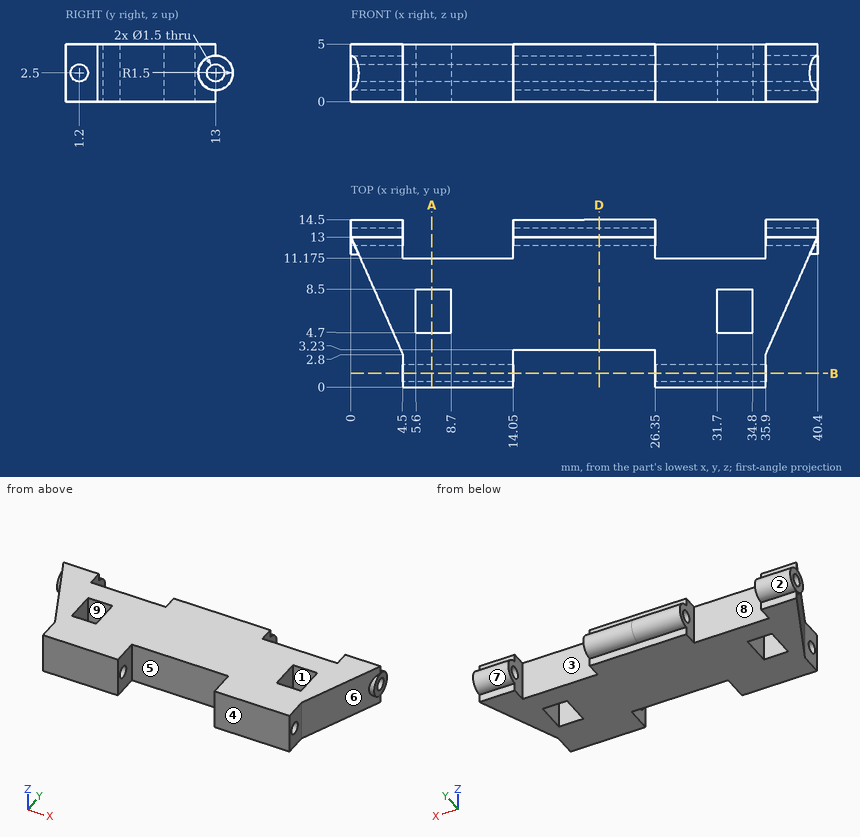
Print and shaded views of the part. All mm, measured from the part's lowest x, y and z. A direction names the side the tool comes from. Round coordinates to 2 decimals unless told otherwise and drop trailing zeros. Write each loop counter-clockwise with the first axis right and the second up, starting at its lowest first coordinate (ties: lowest second). Pieces come first, ordered by that corner, then holes. Notation, with made-up numbers: M 51,70 L 77,70 A21 cw 77,74 Z; hole C 89,33 d4. An arc over 180 degrees is marked long. Use a Markdown table: item, result. Add a question column.
1. Slice it at A-A on x = 7. Give the number of separate pieces and of enclosed holes in the cut face, then the cut area to 3 significant figures.
2. Slice it at D-D on x = 21.5. Give the cut face in (y, z).
3. Drill centre lines: probe 1 along Y at (x, z) = (18.5, 2.5); probe 2 along X at (y, z) = (8, 3.5) (1 decimal); probe 3 along X at (y, z) = (7.75, 4.45) (1 decimal). Where is each one in solid material? Low to high.
4. Slice it at B-B on y = 1.2. Give the cut face in (x, z).
5. 3-axis set-ups, long thin cutter, end or side, ignore diameter. For the marked faces 1, 2, 3, 4 and 5: which of +Z, -Z, +X, -X, +Y, -Y reach the whole face in a straight line?
6. Pull direction X, two halves, no side cores. Call the marked faces 6, 7, 8 and 9: released by +X, released by -X, zero draft, split by the parting line, or undercut.
7. Flat gauge pins, fed straight in: P1, Ø0.9, axis at y = 13, z = 2.5, coming from the +X side; P2, Ø3, axis at y = 7, z = 2, coming from the +X side (1 decimal); P3, Ø0.8, axis at x = 37, z = 4.5, coming from the +Y side; P4, Ø8, axis at x = 12.5, y = 5.5, coming from the -Z side. Where does each tip first touch, or does it go through?
Reply:
| question | item | result |
|---|---|---|
| 1 | separate pieces | 2 |
| 1 | enclosed holes | 1 |
| 1 | area | 35.1 mm^2 |
| 2 | outline | M 3.23,0 L 13,0 L 13,1 A1.5 ccw 13,4 L 13,5 L 3.23,5 Z; hole C 13,2.5 d1.5 |
| 3 | probe 1 | y = 3.23 to 12.25, 13.75 to 14.5 |
| 3 | probe 2 | x = 2.2 to 5.6, 8.7 to 31.7, 34.8 to 38.2 |
| 3 | probe 3 | x = 2.3 to 5.6, 8.7 to 31.7, 34.8 to 38.1 |
| 4 | outline | M 4.5,0 L 14.05,0 L 14.05,1.75 L 4.5,1.75 Z; M 4.5,3.25 L 14.05,3.25 L 14.05,5 L 4.5,5 Z; M 26.35,0 L 35.9,0 L 35.9,1.75 L 26.35,1.75 Z; M 26.35,3.25 L 35.9,3.25 L 35.9,5 L 26.35,5 Z |
| 5 | face 1 | +Z, -Z |
| 5 | face 2 | +X, -X, +Y |
| 5 | face 3 | +Z, -Z, +Y |
| 5 | face 4 | +Z, -Z, +X, -X, -Y |
| 5 | face 5 | +Z, -Z, -Y |
| 6 | face 6 | released by +X |
| 6 | face 7 | zero draft |
| 6 | face 8 | undercut |
| 6 | face 9 | undercut |
| 7 | P1 | passes through |
| 7 | P2 | stops at x = 38.4 |
| 7 | P3 | stops at y = 13 |
| 7 | P4 | stops at z = 0 |
